Could you check a few things on this model? Use its own coordinates, in mm. A direction names the side the tool comes from. Give positions to 0.01 mm unless a question says otherwise; leave off trailing zeros. Order: outer loops, then holes, each group sorted by start corner. A loop starts at its lowest first (then second) coordinate and runs counter-clockwise, first axis right, second up.
(1) Will these pins go through, and if not, where does the flat tip stop? pin 1 (4 mm diameter, centred on y = 2, z = 10, fed in from -X); pin 2 (1 mm diameter, centred on y = 5.5, z = 6, fed in from +X); pin 3 (5 mm diameter, centred on y = 8, z = 10, fed in from +X); pin 4 (0.7 mm diameter, centred on y = 1, z = 9.5, fed in from +X).
(2) If I drill on probe 1 along Z at (x, y) = (0, 2.25); probe 2 along X at (y, z) = (2.25, 8.75); probe 3 along X at (y, z) = (2.25, 1), over which ranges is the centre line in solid material (lowest first)?
(3) Imagine slicing it at B-B, the plane z = 10. Write out the boundary of the cut face in (x, y), then the cut area to 3 significant figures.
(4) If we mould it in two halves opening along Z, with no side actions, what happens to faces 4 (the flat face through (0, 4, 0)), 5 (the flat face through (0, 4, 20)), 6 (the cylindrical face through (-18.294, 6.434, 9.874)), 7 (the flat face through (-2.2, 5, 10.1))? For each: released by +Z, released by -Z, zero draft, split by the parting line, or undercut.
(5) Imagine slicing it at D-D, the plane y = 0.5. State how many separate pieces and enclosed holes the cut face has, then the cut area to 3 significant figures.
(6) Imagine slicing it at A-A, the plane x = 0. Write out the boundary of the cut face in (y, z), then the cut area to 3 significant figures.
(7) On a 3-axis mill with a long thin cutter (end or side, diameter ignored), from which of +Z, -Z, +X, -X, +Y, -Y can I reach the whole of each face in a straight line? I mean faces 1 (the flat face through (18, 0, 10)), 2 (the cylindrical face through (0.651, 6.521, 14.957)), 3 (the flat face through (-9.25, 1, 10)). Say none if no direction works.
(8) Imagine slicing it at C-C, the plane z = 17.25. Write out the boundary of the cut face in (x, y), then the cut area to 3 significant figures.
from build123d import *

# Parameters (mm, degrees)
PAD_DEPTH       = 20
SKETCH001_R     = 5
POCKET_DEPTH    = 4
SKETCH002_R     = 2
POCKET001_DEPTH = 5
FILLET_R        = 1
FILLET001_R     = 1


with BuildPart() as part:
    # Sketch → Pad (new body)
    with BuildSketch(Plane.XY):
        with BuildLine():
            Line((0, 0), (0, 9))
            Line((0, 9), (-12, 9))
            ThreePointArc((-12, 9), (-18.363961, 6.363961), (-21, 0))
            Line((-21, 0), (-14.75, 0))
            Line((-14.75, 0), (-14.75, 2.499989))
            ThreePointArc((-9.25, 2.499989), (-12, 5.25), (-14.75, 2.499989))
            Line((-9.25, 0), (-9.25, 2.499989))
            Line((0, 0), (-9.25, 0))
        make_face()
    extrude(amount=PAD_DEPTH)

    # Mirrored: part across YZ


with BuildPart() as part_1:
    add(part.part)
    add(part.part.mirror(Plane.YZ))

    # Sketch001 (on Face1 of Mirrored) → Pocket (cut)
    with BuildSketch(Plane(origin=(0, 9, 0), x_dir=(-1, 0, 0), z_dir=(0, 1, 0))):
        with Locations((0, 10)):
            Circle(SKETCH001_R)
    extrude(amount=-POCKET_DEPTH, mode=Mode.SUBTRACT)

    # Sketch002 (on Face15 of Pocket) → Pocket001 (cut)
    with BuildSketch(Plane(origin=(0, 5, 0), x_dir=(-1, 0, 0), z_dir=(0, 1, 0))):
        with Locations((0, 10)):
            Circle(SKETCH002_R)
    extrude(amount=-POCKET001_DEPTH, mode=Mode.SUBTRACT)

    # Fillet
    fillet_edges = [part_1.edges().sort_by_distance(p)[0] for p in [
        (-18.363961, 6.363961, 20),
        (-6, 9, 20),
        (6, 9, 20),
        (18.363961, 6.363961, 20),
        (-18.363961, 6.363961, 0),
        (-6, 9, 0),
        (6, 9, 0),
        (18.363961, 6.363961, 0),
    ]]
    fillet(fillet_edges, radius=FILLET_R)

    # Fillet001
    fillet001_edges = [part_1.edges().sort_by_distance(p)[0] for p in [
        (5, 9, 10),
    ]]
    fillet(fillet001_edges, radius=FILLET001_R)


solid = part_1.part
Answer block:
1. pin 1: stops at x = -21
1. pin 2: stops at x = 19.48
1. pin 3: stops at x = 19.12
1. pin 4: stops at x = 20.98
2. probe 1: z = 0 to 8, 12 to 20
2. probe 2: x = -20.71 to -14.75, -9.25 to -1.56, 1.56 to 9.25, 14.75 to 20.71
2. probe 3: x = -20.71 to -14.75, -9.25 to 9.25, 14.75 to 20.71
3. outline: (-21, 0) - (-14.75, 0) - (-14.75, 2.5) arc R2.75 cw to (-9.25, 2.5) - (-9.25, 0) - (-2, 0) - (-2, 5) - (-5, 5) - (-5, 8) arc R1 ccw to (-6, 9) - (-12, 9) arc R9 ccw to start; (2, 0) - (9.25, 0) - (9.25, 2.5) arc R2.75 cw to (14.75, 2.5) - (14.75, 0) - (21, 0) arc R9 ccw to (12, 9) - (6, 9) arc R1 ccw to (5, 8) - (5, 5) - (2, 5) - close
3. area: 232 mm2
4. face 4: released by -Z
4. face 5: released by +Z
4. face 6: zero draft
4. face 7: undercut
5. separate pieces: 3
5. enclosed holes: 1
5. area: 606 mm2
6. outline: (0, 0) - (8, 0) arc R1 ccw to (9, 1) - (9, 4) arc R1 ccw to (8, 5) - (5, 5) - (5, 8) - (0, 8) - close; (0, 12) - (5, 12) - (5, 15) - (8, 15) arc R1 ccw to (9, 16) - (9, 19) arc R1 ccw to (8, 20) - (0, 20) - close
6. area: 119 mm2
7. face 1: +Z, -Z, +X, -X, -Y
7. face 2: +Y
7. face 3: +Z, -Z, -Y
8. outline: (-21, 0) - (-14.75, 0) - (-14.75, 2.5) arc R2.75 cw to (-9.25, 2.5) - (-9.25, 0) - (9.25, 0) - (9.25, 2.5) arc R2.75 cw to (14.75, 2.5) - (14.75, 0) - (21, 0) arc R9 ccw to (12, 9) - (-12, 9) arc R9 ccw to start
8. area: 292 mm2
